Build history of the part. All positions in model axes, mm. A direction names the side the tool comes from. Round coordinates to 2 decimals unless told otherwise and drop trailing zeros. Write each loop counter-clockwise with the first axis right and the second up, starting at its lowest first coordinate (ties: lowest second). Pieces come first, ordered by that corner, then holes.
from build123d import *

# Parameters (mm, degrees)
PAD_DEPTH = 20


with BuildPart() as part:
    # Sketch → Pad (new body, symmetric)
    with BuildSketch(Plane.XZ):
        with BuildLine():
            ThreePointArc((20, 0), (0, 20), (-20, 0))
            Line((-40, 0), (-20, 0))
            Line((-40, -5), (-40, 0))
            Line((-15, -5), (-40, -5))
            Line((-15, 0), (-15, -5))
            ThreePointArc((15, 0), (0, 15), (-15, 0))
            Line((15, 0), (15, -5))
            Line((15, -5), (40, -5))
            Line((40, -5), (40, 0))
            Line((20, 0), (40, 0))
        make_face()
    extrude(amount=PAD_DEPTH, both=True)


solid = part.part
1) Wall check: L1, parallel to X at y = -6.5, z = -1.75; L2, parallel to Z at x = -27, y = 0.5; L3, parallel to X at y = -10, z = 6.25. Give the ranges that are in metal, low to high.
Results:
L1: x = -40 to -15, 15 to 40
L2: z = -5 to 0
L3: x = -19 to -13.64, 13.64 to 19
2) Mould opens along X. For faces 1 (the cylindrical face through (0, 0, 15)), 2 (the cylindrical face through (0, 0, 20)), 3 (the flat face through (-27, 0, -5)), 4 (the flat face through (15, 0, -2)) say: released by +X, released by -X, zero draft, split by the parting line, or undercut.
Results:
face 1: undercut
face 2: split by the parting line
face 3: zero draft
face 4: undercut
3) Slice it at D-D (x = 0). Write the cut outline in (y, z).
Results:
outline: (-20, 15) - (20, 15) - (20, 20) - (-20, 20) - close
4) Slice it at C-C (z = 14). Write the cut outline in (x, y).
Results:
outline: (-14.28, -20) - (-5.39, -20) - (-5.39, 20) - (-14.28, 20) - close; (5.39, -20) - (14.28, -20) - (14.28, 20) - (5.39, 20) - close
5) Pin check, flat tips, straight feed: pin 1 Ø5 at (x, y) = (-2.5, -7.5) entering from -Z; pin 2 Ø8 at (x, y) = (-28, 13) entering from +Z; pin 3 Ø5 at (y, z) = (-2.5, 4) entering from -X. Stop position of each tip, or through.
Results:
pin 1: stops at z = 14.14
pin 2: stops at z = 0
pin 3: stops at x = -19.94
6) Slice it at A-A (z = -1). Write the cut outline in (x, y).
Results:
outline: (-40, -20) - (-15, -20) - (-15, 20) - (-40, 20) - close; (15, -20) - (40, -20) - (40, 20) - (15, 20) - close
7) Slice it at B-B (y = 15.5). Write the cut outline in (x, z).
Results:
outline: (-40, -5) - (-15, -5) - (-15, 0) arc R15 cw to (15, 0) - (15, -5) - (40, -5) - (40, 0) - (20, 0) arc R20 ccw to (-20, 0) - (-40, 0) - close
8) Which spindle directions (+Z, -Z, +X, -X, +Y, -Y) get a long thin tool onto all of the face, cutting with end or side? Do faces 5 (the flat face through (-15, 0, -2)), 6 (the flat face through (-9.1, -20, 12.2)), 7 (the flat face through (-30, 0, 0)), 8 (the flat face through (30, 0, 0)). Say none if no direction does.
Results:
face 5: -Z, +Y, -Y
face 6: +Z, -Z, +X, -X, -Y
face 7: +Z, -X, +Y, -Y
face 8: +Z, +X, +Y, -Y
